Here's how the part is built. I have some questions about the finished solid (model axes, mm). A direction names the side the tool comes from. Round coordinates to 2 decimals unless told otherwise and drop trailing zeros. Order: outer loops, then holes, each group sorted by start corner. A loop starts at its lowest first (then second) coordinate and runs counter-clockwise, first axis right, second up. Notation, with made-up numbers: (-5, 22.5) -> (16, 22.5) arc R19 cw to (16, 49.5) -> close; hole circle Ø10 at (-35, 26). An arc over 180 degrees is marked (long way). One line per item, written item: value.
```python
from build123d import *

# Parameters (mm, degrees)
SKETCH1_R           = 1.6
BOSS_EXTRUDE1_DEPTH = 15
SKETCH2_R           = 3.1
SKETCH2_R_2         = 1.6
BOSS_EXTRUDE2_DEPTH = 1
CHAMFER1_SIZE       = 1


with BuildPart() as part:
    # Sketch1 → Boss-Extrude1 (new body)
    with BuildSketch(Plane(origin=(0, 0, 0), x_dir=(1, 0, 0), z_dir=(0, 1, 0))):
        with BuildLine():
            Line((-1.936491673, -3.5), (1.936491673, -3.5))
            ThreePointArc((1.936491673, -3.5), (4, 0), (1.936491673, 3.5))
            Line((1.936491673, 3.5), (-1.936491673, 3.5))
            ThreePointArc((-1.936491673, 3.5), (-4, 0), (-1.936491673, -3.5))
        make_face()
        with Locations(Location((0, 0, 0), (0, 0, 270))):
            Circle(SKETCH1_R, mode=Mode.SUBTRACT)
    extrude(amount=BOSS_EXTRUDE1_DEPTH)

    # Sketch2 → Boss-Extrude2 (add)
    with BuildSketch(Plane(origin=(0, 15, 0), x_dir=(1, 0, 0), z_dir=(0, 1, 0))):
        with Locations(Location((0, 0, 0), (0, 0, 270))):
            Circle(SKETCH2_R)
        with Locations(Location((0, 0, 0), (0, 0, 270))):
            Circle(SKETCH2_R_2, mode=Mode.SUBTRACT)
    extrude(amount=BOSS_EXTRUDE2_DEPTH)

    # Chamfer1
    chamfer1_edges = [part.edges().sort_by_distance(p)[0] for p in [
        (0, 16, -3.1),
    ]]
    chamfer(chamfer1_edges, length=CHAMFER1_SIZE - 0.0001)  # a hair under: the kernel refuses the full size


solid = part.part
```
Q1. I want a section at C-C on y = 14. Write out the boundary of the cut face in (x, z), then the cut area to 3 significant figures.
Answers:
outline: (-1.94, -3.5) -> (1.94, -3.5) arc R4 ccw to (1.94, 3.5) -> (-1.94, 3.5) arc R4 ccw to start; hole circle Ø3.2 at (0, 0)
area: 39.6 mm2
Q2. I need wall thicknesses on line 1 along Y through (x, z) = (-3.5, -0.75); line 2 along Z through (x, y) = (0.75, 14); line 3 along Z through (x, y) = (-0.5, 15.25). Which ranges of each line are inside material? Lowest first, please.
Answers:
line 1: 0 to 15
line 2: -3.5 to -1.41, 1.41 to 3.5
line 3: -2.81 to -1.52, 1.52 to 2.81
Q3. If we mould it in two halves opening along X, with no side actions, what happens to faces 3 (the face through (0, 7, 3.5)), 4 (the face through (-4, 7, 0)), 5 (the face through (-0.97, 7.89, -1.27)), 6 (the face through (4, 7, 0))? For each: pulls with the +X half, pulls with the -X half, needs draft (parallel to the pull), parting line crosses it, or undercut.
Answers:
face 3: needs draft
face 4: pulls with the -X half
face 5: undercut
face 6: pulls with the +X half
Q4. Which directions (+Z, -Z, +X, -X, +Y, -Y) give clear straight access to the entire face, cutting with the end or side of a thin tool? Please do faces 1 (the face through (0, 7, -3.5)), 2 (the face through (2, 15, -3)).
Answers:
face 1: -Z, +X, -X, +Y, -Y
face 2: +Y
Q5. For P1, Ø2, axis at y = 5.5, z = -1.5, coming from the -X side; P2, Ø1.5, axis at y = 9.5, z = -2.5, coming from the +X side; P3, Ø1, axis at y = 3, z = 1.5, coming from the -X side; P4, Ø1.9, axis at x = 0, z = 0, coming from the -Y side, each with a flat end and sliding along its axis, tell me the tip position at first contact or that it passes through.
Answers:
P1: x = -3.97
P2: x = 3.6
P3: x = -3.87
P4: through
